```python
from build123d import *

# Parameters (mm, degrees)
CROQUIS1_R              = 2.5
CROQUIS1_R_2            = 37.5
CROQUIS1_R_3            = 15
CROQUIS1_R_4            = 2.25
CROQUIS1_W              = 150
CROQUIS1_H              = 150
SALIENTE_EXTRUIR1_DEPTH = 10


with BuildPart() as part:
    # Croquis1 → Saliente-Extruir1 (new body)
    with BuildSketch(Plane.XY):
        with BuildLine():
            Line((15, 0), (435, 0))
            ThreePointArc((435, 0), (445.606601718, 4.393398282), (450, 15))
            Line((450, 15), (450, 235))
            ThreePointArc((450, 235), (445.606601718, 245.606601718), (435, 250))
            Line((435, 250), (15, 250))
            ThreePointArc((15, 250), (4.393398282, 245.606601718), (0, 235))
            Line((0, 235), (0, 15))
            ThreePointArc((0, 15), (4.393398282, 4.393398282), (15, 0))
        make_face()
        with Locations((110, 185.621778265)):
            Circle(CROQUIS1_R, mode=Mode.SUBTRACT)
        with Locations((162.5, 94.689110868)):
            Circle(CROQUIS1_R, mode=Mode.SUBTRACT)
        with Locations((57.5, 94.689110868)):
            Circle(CROQUIS1_R, mode=Mode.SUBTRACT)
        with Locations((110, 125)):
            Circle(CROQUIS1_R_2, mode=Mode.SUBTRACT)
        with Locations((205, 235)):
            Circle(CROQUIS1_R, mode=Mode.SUBTRACT)
        with Locations((245, 235)):
            Circle(CROQUIS1_R, mode=Mode.SUBTRACT)
        with Locations((189.096460098, 45)):
            Circle(CROQUIS1_R_3, mode=Mode.SUBTRACT)
        with Locations((425, 210)):
            Circle(CROQUIS1_R_4, mode=Mode.SUBTRACT)
        with Locations((255, 210)):
            Circle(CROQUIS1_R_4, mode=Mode.SUBTRACT)
        with Locations((255, 40)):
            Circle(CROQUIS1_R_4, mode=Mode.SUBTRACT)
        with Locations((425, 40)):
            Circle(CROQUIS1_R_4, mode=Mode.SUBTRACT)
        with Locations((325, 10)):
            Circle(CROQUIS1_R, mode=Mode.SUBTRACT)
        with Locations((355, 10)):
            Circle(CROQUIS1_R, mode=Mode.SUBTRACT)
        with Locations(Location((95, 10, 0), (0, 0, 180))):
            Circle(CROQUIS1_R, mode=Mode.SUBTRACT)
        with Locations(Location((125, 10, 0), (0, 0, 180))):
            Circle(CROQUIS1_R, mode=Mode.SUBTRACT)
        with Locations((215, 195)):
            Circle(CROQUIS1_R, mode=Mode.SUBTRACT)
        with Locations((235, 195)):
            Circle(CROQUIS1_R, mode=Mode.SUBTRACT)
        with Locations((340, 125)):
            Rectangle(CROQUIS1_W, CROQUIS1_H, mode=Mode.SUBTRACT)
    extrude(amount=SALIENTE_EXTRUIR1_DEPTH)


solid = part.part
```
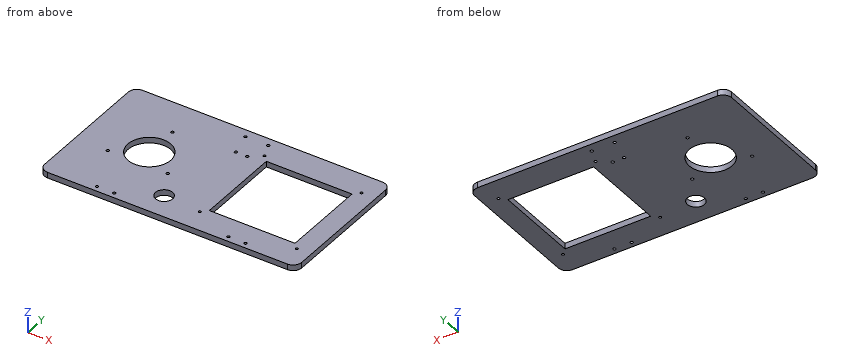
The model under review builds one solid part; all positions refer to its coordinate system, in mm. Round coordinates to 2 decimals unless told otherwise and drop trailing zeros. Write each loop counter-clockwise with the first axis right and the second up, starting at its lowest first coordinate (ties: lowest second). Pieces come first, ordered by that corner, then holes. Notation, with made-up numbers: (73.5, 48) - (103.5, 48) arc R36 cw to (103.5, 83) - close; hole circle Ø8 at (59.25, 18.25). An arc over 180 degrees is marked (long way). One line per question, with ' | ' between items.
Item 1: Add section C-C, the plane y = 155. Give the boundary of the cut face in (x, z).
Resolved:
outline: (0, 0) - (87.5, 0) - (87.5, 10) - (0, 10) - close; (132.5, 0) - (265, 0) - (265, 10) - (132.5, 10) - close; (415, 0) - (450, 0) - (450, 10) - (415, 10) - close
Item 2: To check wall thickness, follow probe 1 along Y at (x, z) = (425, 6.25); probe 2 along Y at (x, z) = (282, 8.5); probe 3 along X at (y, z) = (210, 3.5). State the ranges of each line that lie inside material, in increasing order.
Resolved:
probe 1: y = 0 to 37.75, 42.25 to 207.75, 212.25 to 250 | probe 2: y = 0 to 50, 200 to 250 | probe 3: x = 0 to 252.75, 257.25 to 422.75, 427.25 to 450
Item 3: Add section B-B, the plane y = 125. Give the boundary of the cut face in (x, z), then the cut area to 3 significant figures.
Resolved:
outline: (0, 0) - (72.5, 0) - (72.5, 10) - (0, 10) - close; (147.5, 0) - (265, 0) - (265, 10) - (147.5, 10) - close; (415, 0) - (450, 0) - (450, 10) - (415, 10) - close | area: 2,250 mm2
Item 4: Add section A-A, the plane x = 370.5. Give the boundary of the cut face in (y, z).
Resolved:
outline: (0, 0) - (50, 0) - (50, 10) - (0, 10) - close; (200, 0) - (250, 0) - (250, 10) - (200, 10) - close
